Read the model definition and answer for the solid it produces. Units are mm, in the model's axes. A direction names the side the tool comes from. Give positions to 0.01 mm unless a question says otherwise; leave off trailing zeros. Order: outer loops, then holes, each group sorted by start corner. A loop starts at its lowest first (then second) coordinate and runs counter-clockwise, first axis right, second up. Notation, with made-up numbers: (84, 33.5) -> (90, 33.5) arc R17 ccw to (90, 54.5) -> close; hole circle Ø1 at (25, 7). An arc over 180 degrees is marked (long way). Answer as CSV lines item,"result". Start each with the question number.
1) Straight lines are drawn through the part: L1, parallel to Z at x = -50.8, y = -21.75; L2, parallel to X at y = -17, z = 12 (3 decimals); L3, parallel to Z at x = 8.5, y = -19.5. For each, find the intervals that lie inside material, in ascending order. Write a range as from..to.
2) The mould has two halves that part along X. Classify faces 6 (the face through (60.325, -21, 0)), 7 (the face through (-14, -9.525, -14)), 8 (the face through (-1, -7, 31.75)): +X half, -X half, draft (parallel to the pull), parting line (faces both ways), or undercut.
3) Find section A-A (x = 0). Determine the outline of the cut face in (y, z) (3 decimals).
4) Find section D-D (x = 32). Determine the outline of the cut face in (y, z).
5) Find section C-C (x = 51). Determine the outline of the cut face in (y, z) (3 decimals).
6) Flat-ended cylindrical pins translate along their axes: pin 1 Ø3 at (x, y) = (5, 2.5) entering from +Z; pin 2 Ø10 at (x, z) = (39.5, -25) entering from +Y; pin 3 Ø1.5 at (y, z) = (-1.5, 3.5) entering from +X. Find the tip coordinate at first contact, or state that the pin passes through.
7) Find section B-B (x = -50.8). State how many separate pieces and enclosed holes the cut face has, and give its area (3 significant figures).
8) For faces 1 (the face through (-51, -15.875, 0)), 2 (the face through (46.148, -20.571, -17.619)), 3 (the face through (-28.8, -16.1, 0.4)), 4 (the face through (-15.497, -19.139, -3.441)), 5 (the face through (-7, -25.4, 7)), determine the directions among +Z, -Z, +X, -X, +Y, -Y from which every point of the face is accessible in a straight line to the end or side of a thin tool.
```python
from build123d import *

# Parameters (mm, degrees)
BASE_DEPTH            = 31.75
ROUND_BOSS_DEPTH      = 6.35
ROUND_BOSS_DEPTH_BACK = 25.4
SKETCH2_R             = 15.875
SKETCH3_R             = 9.525
CENTER_HOLE_DEPTH     = 76.201267443
FILLET1_R             = 3.175
CHAMFER1_SIZE         = 2.54
SKETCH4_R             = 4.7625
RIVET_HOLES_DEPTH     = 72.701595171


with BuildPart() as part:
    # Sketch1 → Base (new, symmetric)
    with BuildSketch(Plane.XY):
        with BuildLine():
            Line((0, 0), (-20.139487758, 0))
            ThreePointArc((-20.139487758, 0), (-24.999567349, -0.966729937), (-29.119743879, -3.719743879))
            Line((-29.119743879, -3.719743879), (-40.34506403, -14.94506403))
            ThreePointArc((-40.34506403, -14.94506403), (-41.375108163, -15.633317516), (-42.590128061, -15.875))
            Line((-42.590128061, -15.875), (-60.325, -15.875))
            Line((-60.325, -15.875), (-60.325, -25.4))
            Line((-60.325, -25.4), (-43.360512242, -25.4))
            ThreePointArc((-43.360512242, -25.4), (-38.500432651, -24.433270063), (-34.380256121, -21.680256121))
            Line((-34.380256121, -21.680256121), (-23.15493597, -10.45493597))
            ThreePointArc((-23.15493597, -10.45493597), (-22.124891837, -9.766682484), (-20.909871939, -9.525))
            Line((-20.909871939, -9.525), (0, -9.525))
            Line((0, -9.525), (0, 0))
        make_face()
        with BuildLine():
            Line((20.139487758, 0), (0, 0))
            Line((0, 0), (0, -9.525))
            Line((0, -9.525), (20.909871939, -9.525))
            ThreePointArc((20.909871939, -9.525), (22.124891837, -9.766682484), (23.15493597, -10.45493597))
            Line((23.15493597, -10.45493597), (34.380256121, -21.680256121))
            ThreePointArc((34.380256121, -21.680256121), (38.500432651, -24.433270063), (43.360512242, -25.4))
            Line((43.360512242, -25.4), (60.325, -25.4))
            Line((60.325, -25.4), (60.325, -15.875))
            Line((60.325, -15.875), (42.590128061, -15.875))
            ThreePointArc((42.590128061, -15.875), (41.375108163, -15.633317516), (40.34506403, -14.94506403))
            Line((40.34506403, -14.94506403), (29.119743879, -3.719743879))
            ThreePointArc((29.119743879, -3.719743879), (24.999567349, -0.966729937), (20.139487758, 0))
        make_face()
    extrude(amount=BASE_DEPTH, both=True)

    # Sketch2 → Round Boss (add, two sides: drawn at the far end of the back side and taken through both)
    with BuildSketch(Plane(origin=(0, 0, 0), x_dir=(1, 0, 0), z_dir=(0, 1, 0)).offset(-ROUND_BOSS_DEPTH_BACK)):
        with Locations(Location((0, 0, 0), (0, 0, 270))):
            Circle(SKETCH2_R)
    extrude(amount=ROUND_BOSS_DEPTH + ROUND_BOSS_DEPTH_BACK)

    # Sketch3 → Center Hole (cut, through all)
    with BuildSketch(Plane(origin=(0, 6.35, 0), x_dir=(1, 0, 0), z_dir=(0, 1, 0))):
        with Locations(Location((0, 0, 0), (0, 0, 270))):
            Circle(SKETCH3_R)
    extrude(amount=-CENTER_HOLE_DEPTH, mode=Mode.SUBTRACT)

    # Fillet1
    fillet1_edges = [part.edges().sort_by_distance(p)[0] for p in [
        (0, 0, -15.875),
        (0, -9.525, -15.875),
    ]]
    fillet(fillet1_edges, radius=FILLET1_R)

    # Chamfer1
    chamfer1_edges = [part.edges().sort_by_distance(p)[0] for p in [
        (0, 6.35, -9.525),
    ]]
    chamfer(chamfer1_edges, length=CHAMFER1_SIZE)

    # Sketch4 → Rivet Holes (cut, through all)
    with BuildSketch(Plane(origin=(0, -15.875, 0), x_dir=(1, 0, 0), z_dir=(0, 1, 0))):
        with Locations(Location((-50.8, 19.05, 0), (0, 0, 180))):
            Circle(SKETCH4_R)
        with Locations(Location((-50.8, -19.05, 0), (0, 0, 180))):
            Circle(SKETCH4_R)
        with Locations(Location((50.690390268, -19.05, 0), (0, 0, 180))):
            Circle(SKETCH4_R)
        with Locations(Location((50.690390268, 19.05, 0), (0, 0, 180))):
            Circle(SKETCH4_R)
    extrude(amount=-RIVET_HOLES_DEPTH, mode=Mode.SUBTRACT)


solid = part.part
```
Findings below:
1,L1,"-31.75..-23.81, -14.29..14.29, 23.81..31.75"
1,L2,"-60.325..-29.7, -10.393..10.393, 29.7..60.325"
1,L3,"-13.41..-4.3, 4.3..13.41"
2,face 6,"+X half"
2,face 7,"undercut"
2,face 8,"draft"
3,outline,"(-25.4, -15.875) -> (-12.7, -15.875) arc R3.175 cw to (-9.525, -19.05) -> (-9.525, -31.75) -> (0, -31.75) -> (0, -19.05) arc R3.175 cw to (3.175, -15.875) -> (6.35, -15.875) -> (6.35, -12.065) -> (3.81, -9.525) -> (-25.4, -9.525) -> close; (-25.4, 9.525) -> (3.81, 9.525) -> (6.35, 12.065) -> (6.35, 15.875) -> (3.175, 15.875) arc R3.175 cw to (0, 19.05) -> (0, 31.75) -> (-9.525, 31.75) -> (-9.525, 19.05) arc R3.175 cw to (-12.7, 15.875) -> (-25.4, 15.875) -> close"
4,outline,"(-19.3, -31.75) -> (-6.6, -31.75) -> (-6.6, 31.75) -> (-19.3, 31.75) -> close"
5,outline,"(-25.4, -31.75) -> (-15.875, -31.75) -> (-15.875, -23.802) -> (-25.4, -23.802) -> close; (-25.4, -14.298) -> (-15.875, -14.298) -> (-15.875, 14.298) -> (-25.4, 14.298) -> close; (-25.4, 23.802) -> (-15.875, 23.802) -> (-15.875, 31.75) -> (-25.4, 31.75) -> close"
6,pin 1,"z = 16.04"
6,pin 2,"y = -9.1"
6,pin 3,"x = 27.36"
7,separate pieces,"3"
7,enclosed holes,"0"
7,area,"423 mm²"
8,face 1,"+Z, -Z, -X, +Y"
8,face 2,"+Y, -Y"
8,face 3,"+Z, -Z, -Y"
8,face 4,"-Y"
8,face 5,"+Z, -Z, +X, -X, -Y"
